The figure shows three views and two pictorial views of one solid part (mm, origin at its lowest corner). Answer the questions. Give positions to 0.01 mm unless a question says otherwise; leave off trailing zeros. Loops run counter-clockwise (first coordinate to the right, second up) from the corner with the lowest first, then second, coordinate; pieces in that order, holes last. Notation, with made-up numbers: (-13.75, -18.75) - (11.25, -18.75) arc R24 ccw to (11.25, -1.75) - close; hole circle Ø6 at (6.5, 87.25). An arc over 180 degrees is marked (long way). Write each question's results on one line, items separated by ' | '.
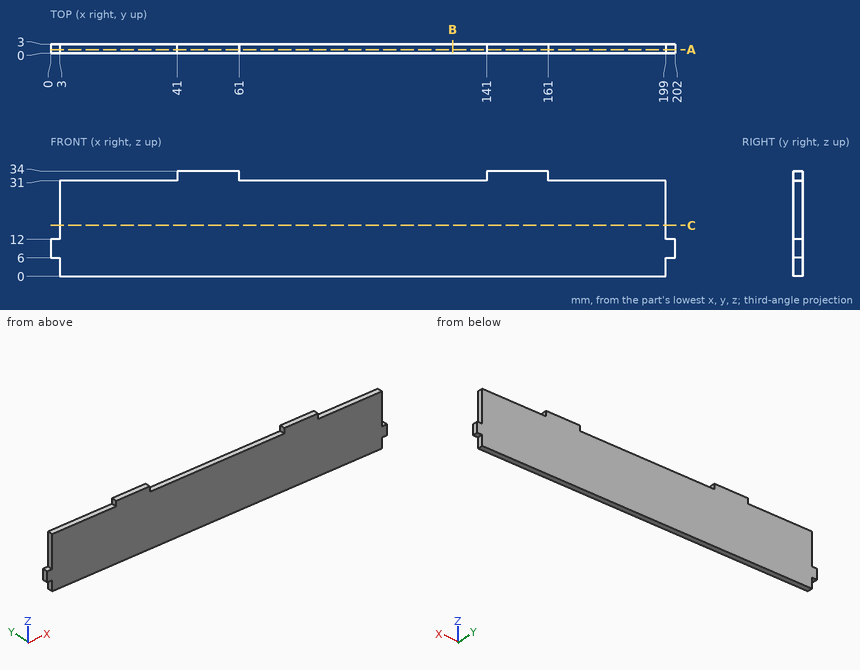
Item 1: A cutting plane is placed at C-C, the plane z = 16.5. Determine the outline of the cut face in (x, y).
Values found:
outline: (3, 0) - (199, 0) - (199, 3) - (3, 3) - close
Item 2: Find the intervals of material crossed by line 1 along Z through (x, y) = (85.5, 2.1); line 2 along X through (y, z) = (2.55, 22.5), in increasing order. Write a range as [from, to].
Values found:
line 1: z = [0, 31] | line 2: x = [3, 199]
Item 3: A cutting plane is placed at B-B, the plane x = 130. Determine the outline of the cut face in (y, z).
Values found:
outline: (0, 0) - (3, 0) - (3, 31) - (0, 31) - close
Item 4: Flat-ended cylindrical pins translate along their axes: P1, Ø0.9, axis at y = 2, z = 32.5, coming from the -X side; P2, Ø1.5, axis at y = 2, z = 32, coming from the +X side; P3, Ø1.5, axis at x = 24.5, y = 1.5, coming from the +Z side. Find the tip coordinate at first contact, or state that the pin passes through.
Values found:
P1: stops at x = 41 | P2: stops at x = 161 | P3: stops at z = 31
Item 5: A cutting plane is placed at A-A, the plane y = 1.2. Determine the outline of the cut face in (x, z).
Values found:
outline: (0, 6) - (3, 6) - (3, 0) - (199, 0) - (199, 6) - (202, 6) - (202, 12) - (199, 12) - (199, 31) - (161, 31) - (161, 34) - (141, 34) - (141, 31) - (61, 31) - (61, 34) - (41, 34) - (41, 31) - (3, 31) - (3, 12) - (0, 12) - close
